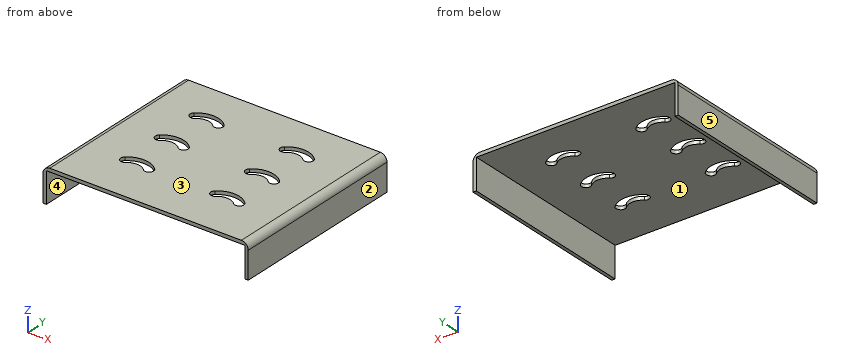
```python
from build123d import *

# Parameters (mm, degrees)
BOSS_EXTRUDE1_DEPTH = 80
FILLET1_R           = 3
CUT_EXTRUDE1_DEPTH  = 1.5


with BuildPart() as part:
    # Sketch1 → Boss-Extrude1 (new body)
    with BuildSketch(Plane(origin=(0, 0, 0), x_dir=(1, 0, 0), z_dir=(0, 1, 0))):
        Polygon((-45.5, 0), (45.5, 0), (45.5, 15.083653846), (44, 15.083653846), (44, 1.5), (-44, 1.5), (-44, 15.083653846), (-45.5, 15.083653846), align=None)
    extrude(amount=BOSS_EXTRUDE1_DEPTH)

    # Fillet1
    fillet1_edges = [part.edges().sort_by_distance(p)[0] for p in [
        (45.5, 40, 0),
        (-45.5, 40, 0),
    ]]
    fillet(fillet1_edges, radius=FILLET1_R)

    # Sketch2 → Cut-Extrude1 (cut)
    with BuildSketch(Plane.XY):
        with BuildLine():
            ThreePointArc((-12.928932188, 62.071067812), (-19.653586872, 64.993998096), (-26.564488849, 62.543705068))
            ThreePointArc((-26.564488849, 62.543705068), (-26.760332093, 59.722066284), (-23.938693309, 59.526223041))
            ThreePointArc((-23.938693309, 59.526223041), (-19.792152123, 60.996398858), (-15.757359313, 59.242640687))
            ThreePointArc((-15.757359313, 59.242640687), (-12.928932188, 59.242640687), (-12.928932188, 62.071067812))
        make_face()
        with BuildLine():
            ThreePointArc((27.071067812, 62.071067812), (20.346413128, 64.993998096), (13.435511151, 62.543705068))
            ThreePointArc((13.435511151, 62.543705068), (13.239667907, 59.722066284), (16.061306691, 59.526223041))
            ThreePointArc((16.061306691, 59.526223041), (20.207847877, 60.996398858), (24.242640687, 59.242640687))
            ThreePointArc((24.242640687, 59.242640687), (27.071067812, 59.242640687), (27.071067812, 62.071067812))
        make_face()
        with BuildLine():
            ThreePointArc((27.071067812, 42.071067812), (20.346413128, 44.993998096), (13.435511151, 42.543705068))
            ThreePointArc((13.435511151, 42.543705068), (13.239667907, 39.722066284), (16.061306691, 39.526223041))
            ThreePointArc((16.061306691, 39.526223041), (20.207847877, 40.996398858), (24.242640687, 39.242640687))
            ThreePointArc((24.242640687, 39.242640687), (27.071067812, 39.242640687), (27.071067812, 42.071067812))
        make_face()
        with BuildLine():
            ThreePointArc((27.071067812, 22.071067812), (20.346413128, 24.993998096), (13.435511151, 22.543705068))
            ThreePointArc((13.435511151, 22.543705068), (13.239667907, 19.722066284), (16.061306691, 19.526223041))
            ThreePointArc((16.061306691, 19.526223041), (20.207847877, 20.996398858), (24.242640687, 19.242640687))
            ThreePointArc((24.242640687, 19.242640687), (27.071067812, 19.242640687), (27.071067812, 22.071067812))
        make_face()
        with BuildLine():
            ThreePointArc((-12.928932188, 42.071067812), (-19.653586872, 44.993998096), (-26.564488849, 42.543705068))
            ThreePointArc((-26.564488849, 42.543705068), (-26.760332093, 39.722066284), (-23.938693309, 39.526223041))
            ThreePointArc((-23.938693309, 39.526223041), (-19.792152123, 40.996398858), (-15.757359313, 39.242640687))
            ThreePointArc((-15.757359313, 39.242640687), (-12.928932188, 39.242640687), (-12.928932188, 42.071067812))
        make_face()
        with BuildLine():
            ThreePointArc((-12.928932188, 22.071067812), (-19.653586872, 24.993998096), (-26.564488849, 22.543705068))
            ThreePointArc((-26.564488849, 22.543705068), (-26.760332093, 19.722066284), (-23.938693309, 19.526223041))
            ThreePointArc((-23.938693309, 19.526223041), (-19.792152123, 20.996398858), (-15.757359313, 19.242640687))
            ThreePointArc((-15.757359313, 19.242640687), (-12.928932188, 19.242640687), (-12.928932188, 22.071067812))
        make_face()
    extrude(amount=-CUT_EXTRUDE1_DEPTH, mode=Mode.SUBTRACT)


solid = part.part
```
The listing builds one solid part. Answer for the finished solid, in the listing's coordinates (mm). Face numbers are marked on the shaded views. A direction names the side the tool comes from. Coordinates: 2 decimals unless noted, no trailing zeros. Loops run counter-clockwise (first coordinate to the right, second up) from the corner with the lowest first, then second, coordinate; pieces in that order, holes last. Notation, with made-up numbers: (69, -25) - (122, -25) arc R20 cw to (122, -1) - close; hole circle Ø4 at (68.25, 34.25). An arc over 180 degrees is marked (long way). Use a Markdown table: item, result. Add a question column.
1) The mould has two halves that part along X. Classify the marked faces 1, 2 and 3: released by +X, released by -X, zero draft, split by the parting line, or undercut.
2) The part is cut by section C-C, the plane y = 10. Give the vertices of the cut face in (x, z).
3) The part is cut by section B-B, the plane x = -21.5. Give the vertices of the cut face in (y, z).
4) Find the intervals of material crossed by line 1 (X direction, y = 32.5, z = -13); line 2 (Z direction, x = -24.5, y = 70.5); line 3 (X direction, y = 47.5, z = -1.75), in increasing order.
5) The part is cut by section A-A, the plane z = -13.75. Give the vertices of the cut face in (x, y).
6) For the marked faces 4 and 5, determine the directions among +Z, -Z, +X, -X, +Y, -Y from which every point of the face is accessible in a straight line to the end or side of a thin tool.
7) The part is cut by section D-D, the plane x = 3. Give the vertices of the cut face in (y, z), and give its area (3 significant figures).
8) Given pin 1 (6 mm diameter, centred on x = 30.5, y = 56.5, fed in from -Z), flat-ended and moving along its own axis, determine where the tip first touches the part or whether it passes through.
Here are the results:
| question | item | result |
|---|---|---|
| 1 | face 1 | undercut |
| 1 | face 2 | released by +X |
| 1 | face 3 | zero draft |
| 2 | outline | (-45.5, -15.08) - (-44, -15.08) - (-44, -1.5) - (44, -1.5) - (44, -15.08) - (45.5, -15.08) - (45.5, -3) arc R3 ccw to (42.5, 0) - (-42.5, 0) arc R3 ccw to (-45.5, -3) - close |
| 3 | outline | (0, -1.5) - (20.81, -1.5) - (20.81, 0) - (0, 0) - close; (24.89, -1.5) - (40.81, -1.5) - (40.81, 0) - (24.89, 0) - close; (44.89, -1.5) - (60.81, -1.5) - (60.81, 0) - (44.89, 0) - close; (64.89, -1.5) - (80, -1.5) - (80, 0) - (64.89, 0) - close |
| 4 | line 1 | x = -45.5 to -44, 44 to 45.5 |
| 4 | line 2 | z = -1.5 to 0 |
| 4 | line 3 | x = -45.23 to -44, 44 to 45.23 |
| 5 | outline | (-45.5, 0) - (-44, 0) - (-44, 80) - (-45.5, 80) - close; (44, 0) - (45.5, 0) - (45.5, 80) - (44, 80) - close |
| 6 | face 4 | -Z, +Y, -Y |
| 6 | face 5 | +Z, -Z, -X, +Y, -Y |
| 7 | outline | (0, -1.5) - (80, -1.5) - (80, 0) - (0, 0) - close |
| 7 | area | 120 mm^2 |
| 8 | pin 1 | stops at z = -1.5 |
